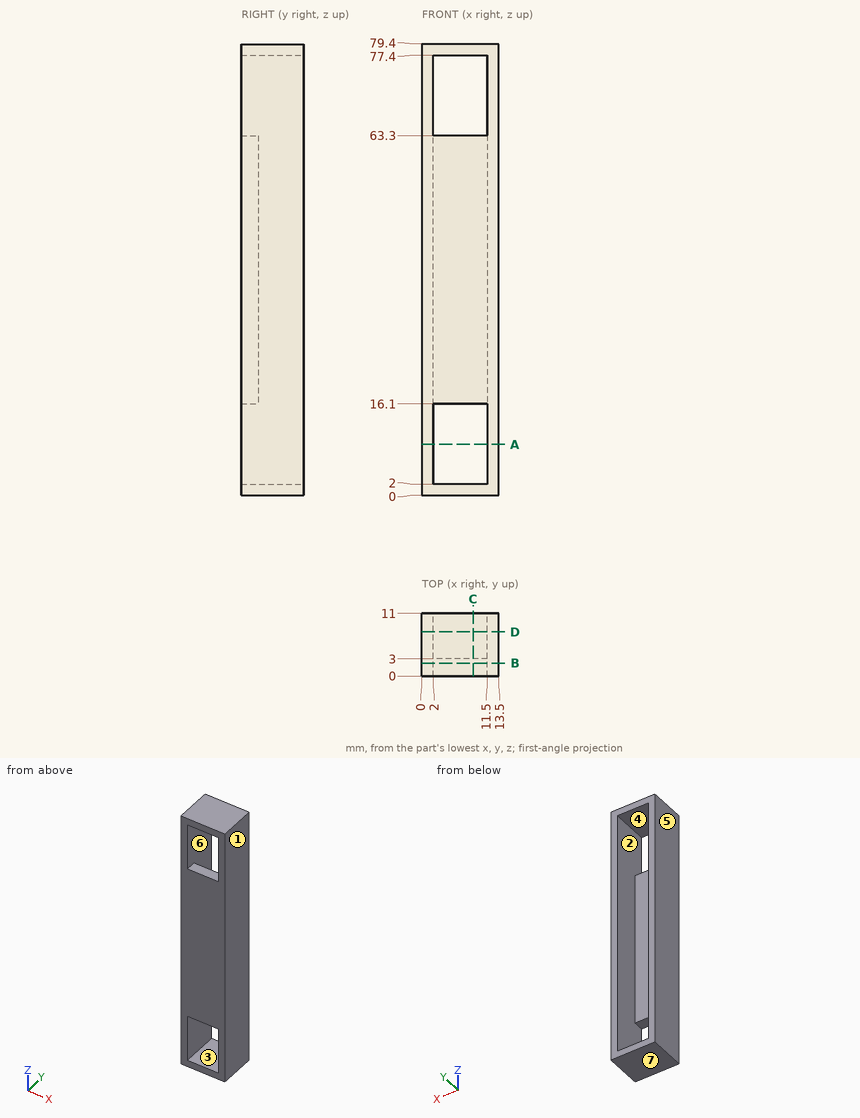
Print and shaded views of the part. All mm, measured from the part's lowest x, y and z. A direction names the side the tool comes from. Round coordinates to 2 decimals unless told otherwise and drop trailing zeros. Write each loop counter-clockwise with the first axis right and the second up, starting at its lowest first coordinate (ties: lowest second). Pieces come first, ordered by that corner, then holes. Notation, with made-up numbers: (-22, 36) -> (18, 36) arc R29 cw to (18, 60) -> close; hole circle Ø8 at (-12, 87). An arc over 180 degrees is marked (long way). Return JSON: item names as keys, results as strings. Group by question number.
Q1. Mould opens along Z. For the marked faces 4, 5, 6 and 7 say: pulls with the +Z half, pulls with the -Z half, needs draft (parallel to the pull), parting line crosses it, or undercut.
Q2. Saw through at A-A on z = 9. Write the cut outline in (x, y).
Q3. Saw through at B-B on y = 2.25. Write the cut outline in (x, z).
Q4. Probe L1, parallel to Z at x = 7.25, y = 1.75; L2, parallel to Z at x = 2.5, y = 4.5; L3, parallel to X at y = 5, z = 50.5. List the from-to ranges inside material, lowest first. Write a range as [from, to].
Q5. Pin check, flat tip, straight feed: pin 1 (3 mm diameter, centred on x = 4.5, z = 32.5, fed in from +Y). Stop position of the tip, or through.
Q6. Saw through at C-C on x = 9. Write the cut outline in (y, z), plus the area to 3 significant figures.
Q7. Saw through at D-D on y = 7.75. Write the cut outline in (x, z), plus the area to 3 significant figures.
Q8. Which spindle directions (+Z, -Z, +X, -X, +Y, -Y) get a long thin tool onto all of the face, cutting with end or side? Do the marked faces 1, 2 and 3. Say none if no direction does.
Answer:
{
 "1": {"face 4": "undercut", "face 5": "needs draft", "face 6": "undercut", "face 7": "pulls with the -Z half"},
 "2": {"outline": "(0, 0) -> (2, 0) -> (2, 11) -> (0, 11) -> close; (11.5, 0) -> (13.5, 0) -> (13.5, 11) -> (11.5, 11) -> close"},
 "3": {"outline": "(0, 0) -> (13.5, 0) -> (13.5, 79.4) -> (0, 79.4) -> close; hole (2, 2) -> (11.5, 2) -> (11.5, 16.1) -> (2, 16.1) -> close; hole (2, 63.3) -> (11.5, 63.3) -> (11.5, 77.4) -> (2, 77.4) -> close"},
 "4": {"L1": "[0, 2], [16.1, 63.3], [77.4, 79.4]", "L2": "[0, 2], [77.4, 79.4]", "L3": "[0, 2], [11.5, 13.5]"},
 "5": {"pin 1": "y = 3"},
 "6": {"outline": "(0, 0) -> (11, 0) -> (11, 2) -> (0, 2) -> close; (0, 16.1) -> (3, 16.1) -> (3, 63.3) -> (0, 63.3) -> close; (0, 77.4) -> (11, 77.4) -> (11, 79.4) -> (0, 79.4) -> close", "area": "186 mm2"},
 "7": {"outline": "(0, 0) -> (13.5, 0) -> (13.5, 79.4) -> (0, 79.4) -> close; hole (2, 2) -> (11.5, 2) -> (11.5, 77.4) -> (2, 77.4) -> close", "area": "356 mm2"},
 "8": {"face 1": "+Z, -Z, +X, +Y, -Y", "face 2": "+Y", "face 3": "+Y, -Y"}
}
